The model under review builds one solid part; all positions refer to its coordinate system, in mm. A direction names the side the tool comes from. Round coordinates to 2 decimals unless told otherwise and drop trailing zeros. Order: outer loops, then holes, each group sorted by start corner. A loop starts at its lowest first (then second) coordinate and runs counter-clockwise, first axis right, second up. Notation, with made-up numbers: M 5,-31 L 17,-31 A32 ccw 17,-4 Z; hole C 28.5,-5.5 d5. An arc over 180 degrees is marked long. Answer as a JSON object with one key per item and string values. Group by question number.
1. Mouldability with a two-part tool opening along X and no side actions: class faces 1 (the face through (-7.96, 1.01, -16.64)), 2 (the face through (-53.061, 1, -9)), 3 (the face through (-10.01, 0.99, -15.55)) as released by +X, released by -X, zero draft, split by the parting line, or undercut.
2. Add section B-B on y = 1.1. Give the number of separate pieces and of enclosed holes in the cut face, and give its area (3 significant figures).
3. Machinability: for faces 4 (the face through (-30, 1, -14.5)), 5 (the face through (-10.01, 0.99, 13.45)), which of the approach directions +Z, -Z, +X, -X, +Y, -Y give a long, thin tool a straight path to every point of the face, cutting with its end or side? Answer none if there is none.
4. Add section C-C on z = -6.5. State the section outline as (x, y) points.
5. Clearance check with flat-ended pins moving along their axes: P1, Ø0.5, axis at y = 0.5, z = -16, coming from the -X side; P2, Ø0.6, axis at x = -29.5, y = 1, coming from the -Z side; P3, Ø1.1, axis at y = 1, z = -16, coming from the +X side (3 decimals); P4, Ø1.3, axis at x = -10.06, z = -14.5, coming from the -Y side. State where each tip first meets the part, or that it passes through.
6. To check wall thickness, follow probe 1 along X at (y, z) = (0.9, 14.5); probe 2 along X at (y, z) = (0.75, 8.7); probe 3 along X at (y, z) = (0.5, -4.5). State the ranges of each line that lie inside material, in increasing order. Write a range as [from, to].
7. Add section A-A on z = 8.7. State the section outline as (x, y) points.
```python
from build123d import *

# Parameters (mm, degrees)
SKETCH1_R           = 1.6
SKETCH1_R_2         = 1.05
BOSS_EXTRUDE1_DEPTH = 2
FILLET1_R           = 3
FILLET2_R           = 1


with BuildPart() as part:
    # Sketch1 → Boss-Extrude1 (new body)
    with BuildSketch(Plane(origin=(0, 0, 0), x_dir=(1, 0, 0), z_dir=(0, 1, 0))):
        Polygon((-27.060616409, 17.5), (-27.060616409, 14.5), (-33.060616409, 14.5), (-33.060616409, 17.5), (-53.060616409, 17.5), (-53.060616409, 0.1), (-60.060616409, 0.1), (-60.060616409, -17.5), (-30.060616409, -17.5), (-0.060616409, -17.5), (-0.060616409, 0.1), (-7.060616409, 0.1), (-7.060616409, 17.5), align=None)
        with Locations(Location((-4.185616409, -8.7, 0), (0, 0, 270))):
            Circle(SKETCH1_R, mode=Mode.SUBTRACT)
        with Locations(Location((-55.935616409, -8.7, 0), (0, 0, 270))):
            Circle(SKETCH1_R, mode=Mode.SUBTRACT)
        with Locations(Location((-10.060616409, -14.5, 0), (0, 0, 270))):
            Circle(SKETCH1_R_2, mode=Mode.SUBTRACT)
        with Locations(Location((-50.060616409, -14.5, 0), (0, 0, 270))):
            Circle(SKETCH1_R_2, mode=Mode.SUBTRACT)
        with Locations(Location((-50.060616409, 14.5, 0), (0, 0, 270))):
            Circle(SKETCH1_R_2, mode=Mode.SUBTRACT)
        with Locations(Location((-10.060616409, 14.5, 0), (0, 0, 270))):
            Circle(SKETCH1_R_2, mode=Mode.SUBTRACT)
    extrude(amount=BOSS_EXTRUDE1_DEPTH)

    # Fillet1
    fillet1_edges = [part.edges().sort_by_distance(p)[0] for p in [
        (-7.060616409, 1, -17.5),
        (-7.060616409, 1, -0.1),
        (-0.060616409, 1, -0.1),
        (-0.060616409, 1, 17.5),
        (-60.060616409, 1, 17.5),
        (-60.060616409, 1, -0.1),
        (-53.060616409, 1, -0.1),
        (-53.060616409, 1, -17.5),
    ]]
    fillet(fillet1_edges, radius=FILLET1_R)

    # Fillet2
    fillet2_edges = [part.edges().sort_by_distance(p)[0] for p in [
        (-33.060616409, 1, -17.5),
        (-33.060616409, 1, -14.5),
        (-27.060616409, 1, -14.5),
        (-27.060616409, 1, -17.5),
    ]]
    fillet(fillet2_edges, radius=FILLET2_R)


solid = part.part
```
Recorded:
{
 "1": {"face 1": "released by +X", "face 2": "released by -X", "face 3": "undercut"},
 "2": {"separate pieces": "1", "enclosed holes": "6", "area": "1,800 mm²"},
 "3": {"face 4": "-Z, +Y, -Y", "face 5": "+Y, -Y"},
 "4": {"outline": "M -53.06,0 L -7.06,0 L -7.06,2 L -53.06,2 Z"},
 "5": {"P1": "stops at x = -52.79", "P2": "stops at z = -14.5", "P3": "stops at x = -7.215", "P4": "passes through"},
 "6": {"probe 1": "x = [-60.06, -51.11], [-49.01, -11.11], [-9.01, -0.06]", "probe 2": "x = [-60.06, -57.54], [-54.34, -5.79], [-2.59, -0.06]", "probe 3": "x = [-53.06, -7.06]"},
 "7": {"outline": "M -60.06,0 L -57.54,0 L -57.54,2 L -60.06,2 Z; M -54.34,0 L -5.79,0 L -5.79,2 L -54.34,2 Z; M -2.59,0 L -0.06,0 L -0.06,2 L -2.59,2 Z"}
}
